Read the model definition and answer for the solid it produces. Units are mm, in the model's axes. Face numbers are marked on the shaded views. Coordinates: 2 decimals unless noted, no trailing zeros. Write each loop counter-clockwise with the first axis right and the second up, starting at its lowest first coordinate (ties: lowest second). Pieces come first, ordered by that corner, then holes. Notation, with made-up numbers: (-36, 13) -> (14, 13) arc R15 ccw to (14, 27) -> close; hole circle Ø1 at (-4, 73). An arc over 180 degrees is marked (long way). Return JSON: item names as keys, results as strings.
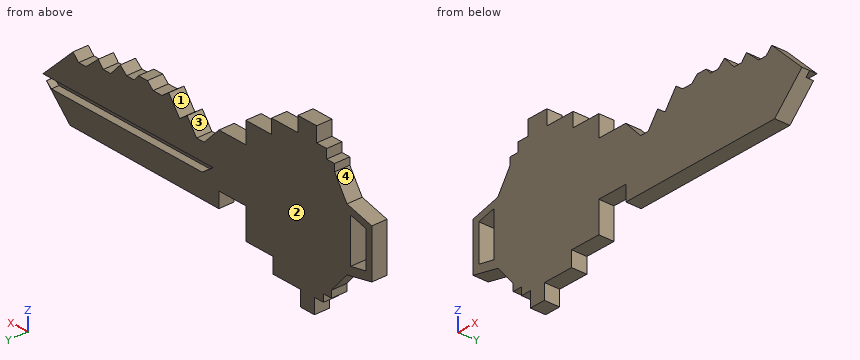
from build123d import *

# Parameters (mm, degrees)
F2_DEPTH = 1.5875
F4_DEPTH = 1.5875
F5_DEPTH = 0.79375


with BuildPart() as f2:
    # F0 (on Front) → F2 (new body)
    with BuildSketch(Plane.XZ):
        Polygon((9.796584, 23.349988), (9.796584, 21.762488), (27.18009, 21.868323), (30.369195, 25.123497), (26.843533, 28.5776), (26.180675, 27.901009), (25.318117, 27.901009), (23.894507, 29.16527), (23.305416, 28.501929), (22.430886, 28.501929), (21.314058, 29.752675), (20.577589, 29.095061), (19.692793, 29.095061), (19.176317, 29.681733), (18.144356, 29.681733), (17.481392, 29.075808), (16.444386, 29.075808), (15.645858, 29.650049), (14.37626, 27.884573), (13.501141, 28.513893), (12.396776, 26.978187), (11.511933, 26.978187), (9.777895, 28.805975), (6.630678, 28.805975), (6.630678, 31.001708), (3.629841, 31.001708), (3.629841, 32.465532), (0.555814, 32.465532), (0.555814, 34.002542), (-1.63992, 34.002542), (-1.63992, 32.465532), (-2.810978, 32.465532), (-2.810978, 31.514045), (-3.735324, 31.514045), (-3.735324, 30.767458), (-5.180371, 28.516009), (-5.180371, 22.166009), (-3.396362, 20.060986), (-3.375214, 19.322162), (-2.425008, 19.322162), (-2.425008, 18.557757), (-1.376822, 18.557757), (-1.376822, 16.999988), (0.271584, 16.999988), (0.271584, 18.587488), (3.446584, 18.587488), (3.446584, 20.174988), (6.621584, 20.174988), (6.621584, 23.349988), align=None)
        Polygon((-8.077298, 22.759162), (-5.180371, 22.166009), (-5.180371, 28.516009), (-8.077298, 27.770618), (-8.077298, 27.149362), align=None)
    extrude(amount=F2_DEPTH)

    # F3 (on face) → F4 (cut)
    with BuildSketch(Plane.XZ.offset(1.5875)):
        Polygon((-5.609657, 27.647099), (-5.833327, 27.652194), (-7.391887, 27.251171), (-7.391887, 23.460561), (-5.609657, 23.115788), align=None)
    extrude(amount=-F4_DEPTH, mode=Mode.SUBTRACT)

    # F1 (on face) → F5 (cut)
    with BuildSketch(Plane.XZ):
        Polygon((30.482488, 25.144005), (28.022444, 25.144005), (10.450701, 25.144005), (11.739296, 24.206847), (29.369611, 24.206847), align=None)
    extrude(amount=F5_DEPTH, mode=Mode.SUBTRACT)


solid = f2.part
1. The part is cut by section B-B (z = 18). Determine the outline of the cut face in (x, y).
Taken from the geometry:
{"outline": "(-1.38, -1.59) -> (0.27, -1.59) -> (0.27, 0) -> (-1.38, 0) -> close"}
2. For a pull along X with two mould halves and no side action, classify the marked faces 1, 2, 3 and 4 as +X half, -X half, draft (parallel to the pull), parting line (faces both ways), or undercut.
Taken from the geometry:
{"face 1": "undercut", "face 2": "draft", "face 3": "undercut", "face 4": "-X half"}
3. Flat-ended cylindrical pins translate along their axes: pin 1 Ø0.8 at (x, y) = (1.5, -1) entering from -Z; pin 2 Ø0.8 at (y, z) = (-1, 33.5) entering from -X; pin 3 Ø0.5 at (y, z) = (-1, 32) entering from -X. Find the tip coordinate at first contact, or state that the pin passes through.
Taken from the geometry:
{"pin 1": "stops at z = 18.59", "pin 2": "stops at x = -1.64", "pin 3": "stops at x = -2.81"}
4. The part is cut by section D-D (x = 28). Determine the outline of the cut face in (y, z), then the cut area to 3 significant figures.
Taken from the geometry:
{"outline": "(-1.59, 22.71) -> (0, 22.71) -> (0, 24.21) -> (-0.79, 24.21) -> (-0.79, 25.14) -> (0, 25.14) -> (0, 27.44) -> (-1.59, 27.44) -> close", "area": "6.78 mm2"}
5. The part is cut by section C-C (z = 32). Determine the outline of the cut face in (x, y), then the cut area to 3 significant figures.
Taken from the geometry:
{"outline": "(-2.81, -1.59) -> (3.63, -1.59) -> (3.63, 0) -> (-2.81, 0) -> close", "area": "10.2 mm2"}
6. Consider L1, parallel to X at y = -0.7, z = 19 (3 decimals); L2, parallel to X at y = -1.5, z = 32.5; L3, parallel to Z at x = 3, y = -0.75. Determine where each line is inside the solid, lowest interval first.
Taken from the geometry:
{"L1": "x = -2.425 to 3.447", "L2": "x = -1.64 to 0.56", "L3": "z = 18.59 to 32.47"}
7. The part is cut by section A-A (x = 13). Determine the outline of the cut face in (y, z), then the cut area to 3 significant figures.
Taken from the geometry:
{"outline": "(-1.59, 21.78) -> (0, 21.78) -> (0, 24.21) -> (-0.79, 24.21) -> (-0.79, 25.14) -> (0, 25.14) -> (0, 27.82) -> (-1.59, 27.82) -> close", "area": "8.84 mm2"}
